Read the model definition and answer for the solid it produces. Units are mm, in the model's axes. Face numbers are marked on the shaded views. A direction names the side the tool comes from. Give positions to 0.01 mm unless a question says otherwise; leave off trailing zeros. Loops run counter-clockwise (first coordinate to the right, second up) from the corner with the lowest first, then second, coordinate; pieces in that order, holes last. Notation, with made-up numbers: (16, -29) - (64, -29) arc R14 ccw to (64, -2) - close; hole circle Ø9 at (1, -35). An arc over 180 degrees is marked (long way). Write item = value, one per line.
```python
from build123d import *

# Parameters (mm, degrees)
BOSS_EXTRUDE1_DEPTH   = 3
BOSS_EXTRUDE2_DEPTH   = 3.5
BOSS_EXTRUDE3_DEPTH   = 3.7
SKETCH4_R             = 2.88
BOSS_EXTRUDE4_DEPTH   = 12
SKETCH11_W            = 6.5
SKETCH11_H            = 0.7
CUT_EXTRUDE3_DEPTH    = 23
F_2_5MM_DOWEL_HOLE1_D = 2.5
SKETCH8_R             = 1.35
CUT_EXTRUDE1_DEPTH    = 38.747052924
FILLET1_R             = 1
FILLET2_R             = 1
CUT_EXTRUDE2_START    = -8
CUT_EXTRUDE2_DEPTH    = 8
FILLET3_R             = 0.5


with BuildPart() as part:
    # Sketch1 → Boss-Extrude1 (new body)
    with BuildSketch(Plane(origin=(0, 0, 0), x_dir=(1, 0, 0), z_dir=(0, 1, 0))):
        with BuildLine():
            Line((0, 13), (16, 13))
            Line((16, 13), (16, 7))
            Line((16, 7), (0, 7))
            ThreePointArc((0, 7), (-7, 0), (0, -7))
            Line((0, -7), (16, -7))
            Line((16, -7), (16, -13))
            Line((16, -13), (0, -13))
            ThreePointArc((0, -13), (-13, 0), (0, 13))
        make_face()
    extrude(amount=BOSS_EXTRUDE1_DEPTH)

    # Sketch2 → Boss-Extrude2 (add)
    with BuildSketch(Plane(origin=(0, 3, 0), x_dir=(1, 0, 0), z_dir=(0, 1, 0))):
        with BuildLine():
            Line((0, 13), (16, 13))
            Line((16, 13), (16, 10))
            Line((16, 10), (0, 10))
            ThreePointArc((0, 10), (-10, 0), (0, -10))
            Line((0, -10), (16, -10))
            Line((16, -10), (16, -13))
            Line((16, -13), (0, -13))
            ThreePointArc((0, -13), (-13, 0), (0, 13))
        make_face()
    extrude(amount=BOSS_EXTRUDE2_DEPTH)

    # Sketch3 → Boss-Extrude3 (add)
    with BuildSketch(Plane(origin=(0, 6.5, 0), x_dir=(1, 0, 0), z_dir=(0, 1, 0))):
        with BuildLine():
            Line((16, 13), (0, 13))
            ThreePointArc((0, 13), (-13, 0), (0, -13))
            Line((0, -13), (16, -13))
            Line((16, -13), (16, -7))
            Line((16, -7), (16, 7))
            Line((16, 7), (16, 13))
        make_face()
    extrude(amount=BOSS_EXTRUDE3_DEPTH)

    # Sketch4 → Boss-Extrude4 (add)
    with BuildSketch(Plane(origin=(0, 10.2, 0), x_dir=(1, 0, 0), z_dir=(0, 1, 0))):
        with Locations(Location((0, 0, 0), (0, 0, 270))):
            Circle(SKETCH4_R)
    extrude(amount=BOSS_EXTRUDE4_DEPTH)

    # Sketch11 → Cut-Extrude3 (cut)
    with BuildSketch(Plane(origin=(16, 0, 0), x_dir=(0, 0, -1), z_dir=(1, 0, 0))):
        with Locations((0, 6.85)):
            Rectangle(SKETCH11_W, SKETCH11_H)
    extrude(amount=-CUT_EXTRUDE3_DEPTH, mode=Mode.SUBTRACT)

    # Ø2.5mm Dowel Hole1 (through all)
    with Locations(Plane(origin=(-0.002429038, 18.104937254, 2.879998976), x_dir=(0.999999644325, 0, 0.000843415861), z_dir=(-0.000843415861, 0, 0.999999644325))):
        with Locations((0, 0)):
            Hole(F_2_5MM_DOWEL_HOLE1_D / 2)

    # Sketch8 → Cut-Extrude1 (cut, through all)
    with BuildSketch(Plane.XY.offset(13)):
        with Locations((12.5, 5.1)):
            Circle(SKETCH8_R)
    extrude(amount=-CUT_EXTRUDE1_DEPTH, mode=Mode.SUBTRACT)

    # Fillet1
    fillet1_edges = [part.edges().sort_by_distance(p)[0] for p in [
        (8, 0, -13),
        (8, 0, -7),
        (-7, 0, 0),
        (16, 5.1, 13),
        (-13, 10.2, 0),
        (8, 10.2, 13),
        (8, 10.2, -13),
        (8, 0, 7),
        (8, 0, 13),
        (-13, 0, 0),
    ]]
    fillet(fillet1_edges, radius=FILLET1_R)

    # Fillet2
    fillet2_edges = [part.edges().sort_by_distance(p)[0] for p in [
        (0, 10.2, -2.88),
    ]]
    fillet(fillet2_edges, radius=FILLET2_R)

    # Sketch10 → Cut-Extrude2 (cut)
    with BuildSketch(Plane(origin=(0, 22.2, 0), x_dir=(1, 0, 0), z_dir=(0, 1, 0)).offset(CUT_EXTRUDE2_START)):
        with BuildLine():
            Line((-2.793635624, 0.7), (2.793635624, 0.7))
            ThreePointArc((2.793635624, 0.7), (2.88, 0), (2.793635624, -0.7))
            Line((2.793635624, -0.7), (-2.793635624, -0.7))
            ThreePointArc((-2.793635624, -0.7), (-2.88, 0), (-2.793635624, 0.7))
        make_face()
    extrude(amount=CUT_EXTRUDE2_DEPTH, mode=Mode.SUBTRACT)

    # Fillet3
    fillet3_edges = [part.edges().sort_by_distance(p)[0] for p in [
        (0, 22.2, -2.88),
        (1.771778767, 22.2, 2.270506551),
    ]]
    fillet(fillet3_edges, radius=FILLET3_R)


solid = part.part
```
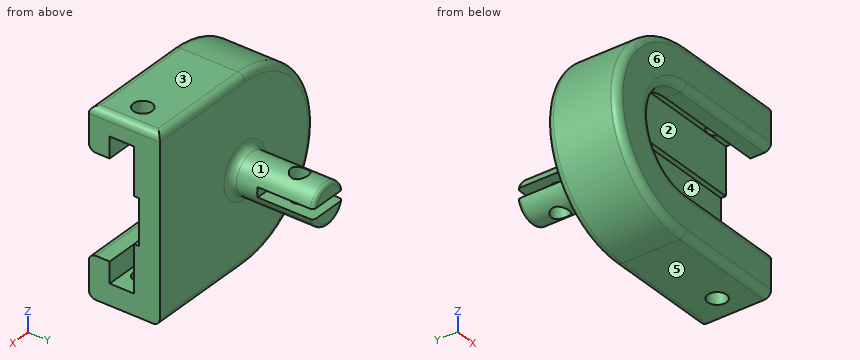
1) A cutting plane is placed at A-A on y = 5.1. Determine the outline of the cut face in (x, z), then the cut area to 3 significant figures.
Output:
outline = (0, -13) - (11.15, -13) - (11.15, -10) - (0, -10) arc R10 cw to (0, 10) - (11.15, 10) - (11.15, 13) - (0, 13) arc R13 ccw to start; (13.85, -13) - (16, -13) - (16, -10) - (13.85, -10) - close; (13.85, 10) - (16, 10) - (16, 12) arc R1 ccw to (15, 13) - (13.85, 13) - close
area = 188 mm²
2) Each of these flat-tipped pins is pushed along its axis until it touches: P1, Ø4.5, axis at x = -1, y = 19.5, coming from the +Z side; P2, Ø3, axis at y = 6, z = 6, coming from the -X side; P3, Ø2, axis at x = 12.5, y = 5.1, coming from the -Z side; P4, Ø10, axis at x = 9, z = 1, coming from the +Y side. Where does it stop, or does it pass through?
Output:
P1 = 2.88
P2 = -12.2
P3 = through
P4 = 10.2
3) Find the intervals of material crossed by probe 1 along Z at (x, y) = (9.5, 6); probe 2 along Y at (x, z) = (12.5, -11); probe 3 along Y at (x, z) = (13, 9), in increasing order.
Output:
probe_1 = -13 to -10, 10 to 13
probe_2 = 0 to 3.75, 6.45 to 10.2
probe_3 = 0 to 3, 6.5 to 10.2
4) The mould has two halves that part along Z. Classify the marked faces 4, 5 and 6: pulls with the +Z half, pulls with the -Z half, needs draft (parallel to the pull), parting line crosses it, or undercut.
Output:
face_4 = undercut
face_5 = pulls with the -Z half
face_6 = needs draft
5) A cutting plane is placed at B-B on x = 12.5. Give the number of separate pieces and of enclosed holes in the cut face, then the cut area to 3 significant figures.
Output:
separate_pieces = 3
enclosed_holes = 0
area = 131 mm²
6) A cutting plane is placed at C-C on z = 0. Determine the outline of the cut face in (x, y), then the cut area to 3 significant figures.
Output:
outline = (-13, 1) arc R1 ccw to (-12, 0) - (-8, 0) arc R1 ccw to (-7, 1) - (-7, 3) - (-10, 3) - (-10, 6.5) - (-7, 6.5) - (-7, 7.2) - (16, 7.2) - (16, 10.2) - (3.88, 10.2) arc R1 cw to (2.88, 11.2) - (2.88, 14.2) - (-2.88, 14.2) - (-2.88, 11.2) arc R1 cw to (-3.88, 10.2) - (-12, 10.2) arc R1 ccw to (-13, 9.2) - close
area = 143 mm²
7) A cutting plane is placed at D-D on y = 21. Determine the outline of the cut face in (x, z), then the cut area to 3 significant figures.
Output:
outline = (-2.79, -0.7) arc R2.88 ccw to (2.79, -0.7) - close; (-2.79, 0.7) - (2.79, 0.7) arc R2.88 ccw to start
area = 18.1 mm²
8) A tool of negligible diameter and unlimited length cuts with its end or side. For the marked faces 1, 2 and 3, from which of +Z, -Z, +X, -X, +Y, -Y can it reach the whole face along a straight path? Write none if from no direction.
Output:
face_1 = +Y
face_2 = +X
face_3 = +Z, +X, -X, +Y, -Y
